Can you work these out from the model? Positions are in its coordinate system, mm. Face numbers are marked on the shaded views. A direction names the side the tool comes from. Coordinates: 2 decimals unless noted, no trailing zeros. Order: outer loops, then holes, each group sorted by start corner. A loop starts at its lowest first (then second) coordinate and runs counter-clockwise, first axis right, second up.
```python
from build123d import *

# Parameters (mm, degrees)
SKETCH1_W            = 100
SKETCH1_H            = 20
BOSS_EXTRUDE1_DEPTH  = 3
BOSS_EXTRUDE3_DEPTH  = 20
SKETCH8_W            = 24
SKETCH8_H            = 3
BOSS_EXTRUDE6_DEPTH  = 20
SKETCH10_W           = 6
SKETCH10_H           = 3
BOSS_EXTRUDE9_DEPTH  = 20
SKETCH12_R           = 1.6
CUT_EXTRUDE1_DEPTH   = 80
SKETCH11_R           = 1.5
CUT_EXTRUDE2_DEPTH   = 20
SKETCH13_W           = 7.961309781
SKETCH13_H           = 15.301040779
BOSS_EXTRUDE10_DEPTH = 3


with BuildPart() as part:
    # Sketch1 → Boss-Extrude1 (new body)
    with BuildSketch(Plane(origin=(0, 0, 0), x_dir=(1, 0, 0), z_dir=(0, 1, 0))):
        with Locations((50, 10)):
            Rectangle(SKETCH1_W, SKETCH1_H)
    extrude(amount=BOSS_EXTRUDE1_DEPTH)

    # Sketch4 → Boss-Extrude3 (add)
    with BuildSketch(Plane(origin=(0, 0, -20), x_dir=(-1, 0, 0), z_dir=(0, 0, -1))):
        Polygon((0, -43), (0, 0), (-3, 0), (-3, -24), (-3, -26.692100843), (-3, -43), align=None)
    extrude(amount=-BOSS_EXTRUDE3_DEPTH)

    # Sketch8 → Boss-Extrude6 (add)
    with BuildSketch(Plane(origin=(0, 0, -20), x_dir=(-1, 0, 0), z_dir=(0, 0, -1))):
        with Locations((-12, -41.5)):
            Rectangle(SKETCH8_W, SKETCH8_H)
    extrude(amount=-BOSS_EXTRUDE6_DEPTH)

    # Sketch10 → Boss-Extrude9 (add)
    with BuildSketch(Plane.XY):
        with Locations((5.126533602, -28.13)):
            Rectangle(SKETCH10_W, SKETCH10_H)
    extrude(amount=-BOSS_EXTRUDE9_DEPTH)

    # Sketch12 → Cut-Extrude1 (cut)
    with BuildSketch(Plane(origin=(0, -43, 0), x_dir=(-1, 0, 0), z_dir=(0, -1, 0))):
        with Locations(Location((-10.38, 5.6, 0), (0, 0, 90))):
            Circle(SKETCH12_R)
        with Locations(Location((-10.38, 15.6, 0), (0, 0, 90))):
            Circle(SKETCH12_R)
    extrude(amount=-CUT_EXTRUDE1_DEPTH, mode=Mode.SUBTRACT)

    # Sketch11 → Cut-Extrude2 (cut)
    with BuildSketch(Plane.XZ.offset(43)):
        with Locations(Location((20.852680531, -10.165848845, 0), (0, 0, 270))):
            Circle(SKETCH11_R)
    extrude(amount=-CUT_EXTRUDE2_DEPTH, mode=Mode.SUBTRACT)

    # Sketch13 → Boss-Extrude10 (add)
    with BuildSketch(Plane.XZ.offset(43)):
        with Locations((9.051384729, -11.125007192)):
            Rectangle(SKETCH13_W, SKETCH13_H)
    extrude(amount=-BOSS_EXTRUDE10_DEPTH)


solid = part.part
```
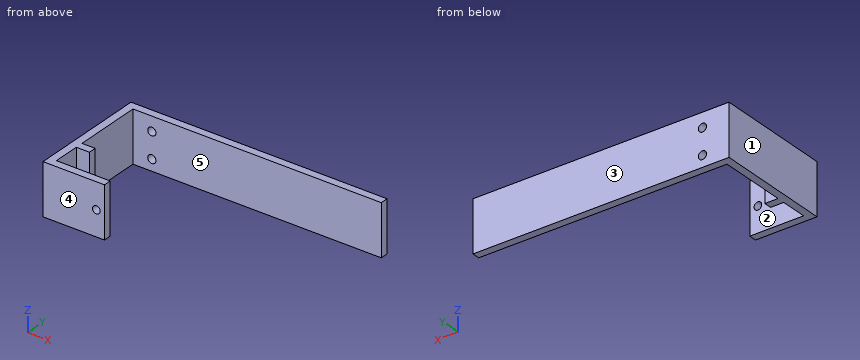
1. Please list where these lines run through material, in increasing order: probe 1 along Y at (x, z) = (7.5, -15.25); probe 2 along Y at (x, z) = (23, -5); probe 3 along X at (y, z) = (1.4, -15.6).
Completed:
probe 1: y = -43 to -40, -29.63 to -26.63, 0 to 3
probe 2: y = -43 to -40, 0 to 3
probe 3: x = 0 to 8.78, 11.98 to 100
2. Imagine slicing it at B-B on z = -15.6. Please give me the cut outline in (x, y), then the cut area to 3 significant figures.
Completed:
outline: (0, -43) - (24, -43) - (24, -40) - (3, -40) - (3, -29.63) - (8.13, -29.63) - (8.13, -26.63) - (3, -26.63) - (3, 0) - (8.78, 0) - (8.78, 3) - (0, 3) - close; (11.98, 0) - (100, 0) - (100, 3) - (11.98, 3) - close
area: 498 mm2
3. Imagine slicing it at D-D on y = -37. Please give me the cut outline in (x, z), then the cut area to 3 significant figures.
Completed:
outline: (0, -20) - (3, -20) - (3, 0) - (0, 0) - close
area: 60.0 mm2
4. On a 3-axis mill with a long thin cutter (end or side, diameter ignored), from which of +Z, -Z, +X, -X, +Y, -Y can I reach the whole of each face in a straight line? I mean the marked faces 4 and 5. Say none if no direction works.
Completed:
face 4: +Z, -Z, +X, -X, -Y
face 5: +Z, -Z, +X
5. Thinking about a two-plate mould opening in Y: for the marked faces 1, 2 and 3, which applies, pulls with the +Y half, pulls with the -Y half, needs draft (parallel to the pull), parting line crosses it, or undercut?
Completed:
face 1: needs draft
face 2: undercut
face 3: pulls with the +Y half
6. I'm going to push flat-ended pins straight in: pin 1 (5 mm diameter, centred on y = -35.5, z = -6.5, fed in from +X); pin 2 (6 mm diameter, centred on y = -32, z = -16.5, fed in from +X); pin 3 (2.5 mm diameter, centred on x = 20.85, z = -10.17, fed in from -Y); pin 4 (1 mm diameter, centred on x = 50, y = -2, fed in from +Z). Where does each tip first touch, or does it pass through?
Completed:
pin 1: stops at x = 3
pin 2: stops at x = 8.13
pin 3: stops at y = 0
pin 4: passes through
7. Imagine slicing it at A-A on x = 10.38. Please give me the cut outline in (y, z), then the cut area to 3 significant figures.
Completed:
outline: (-43, -20) - (-40, -20) - (-40, 0) - (-43, 0) - close; (0, -20) - (3, -20) - (3, -17.2) - (0, -17.2) - close; (0, -14) - (3, -14) - (3, -7.2) - (0, -7.2) - close; (0, -4) - (3, -4) - (3, 0) - (0, 0) - close
area: 101 mm2
